from build123d import *

# Parameters (mm, degrees)
SKETCH_1_R      = 1.59
EXTRUDE_1_DEPTH = 1


with BuildPart() as part:
    # Эскиз1 → Бобышка-Вытянуть1 (new body)
    with BuildSketch(Plane(origin=(0, 0, 0), x_dir=(1, 0, 0), z_dir=(0, 1, 0))):
        with BuildLine():
            Line((-45.084998549, -11.549999236), (-45.084998549, -45.944999694))
            ThreePointArc((-45.084998549, -45.944999694), (-44.499026016, -47.35966253), (-43.084363181, -47.945635063))
            Line((-43.084363181, -47.945635063), (-11.549432233, -47.945635063))
            ThreePointArc((-11.549432233, -47.945635063), (-10.700904348, -47.594163453), (-10.349432233, -46.745635778))
            ThreePointArc((-10.349432233, -46.745635778), (-9.997959671, -45.897107024), (-9.149430707, -45.545634967))
            Line((-9.149430707, -45.545634967), (9.15056853, -45.545634967))
            ThreePointArc((9.15056853, -45.545634967), (9.999097494, -45.897107024), (10.350570056, -46.745635778))
            ThreePointArc((10.350570056, -46.745635778), (10.702042171, -47.594163453), (11.550570056, -47.945635063))
            Line((11.550570056, -47.945635063), (43.085566089, -47.945635063))
            ThreePointArc((43.085566089, -47.945635063), (44.499379352, -47.360014435), (45.08499998, -45.946201172))
            Line((45.08499998, -45.946201172), (45.08499998, -11.550001001))
            ThreePointArc((45.08499998, -11.550001001), (44.73352809, -10.70147331), (43.885000099, -10.350002145))
            ThreePointArc((43.885000099, -10.350002145), (43.03647086, -9.998530464), (42.684998454, -9.150001525))
            Line((42.684998454, -9.150001525), (42.684998454, 9.150001525))
            ThreePointArc((42.684998454, 9.150001525), (43.03647086, 9.998530464), (43.885000099, 10.350002145))
            ThreePointArc((43.885000099, 10.350002145), (44.733527178, 10.701472863), (45.08499962, 11.549999228))
            Line((45.08499962, 11.549999228), (45.08499962, 45.944999694))
            ThreePointArc((45.08499962, 45.944999694), (44.499213182, 47.359213257), (43.08499962, 47.944999694))
            Line((43.08499962, 47.944999694), (11.549999772, 47.944999694))
            ThreePointArc((11.549999772, 47.944999694), (10.701471635, 47.593527832), (10.349999772, 46.744999694))
            ThreePointArc((10.349999772, 46.744999694), (9.998527463, 45.896470478), (9.149998246, 45.544998168))
            Line((9.149998246, 45.544998168), (-9.149997176, 45.544998168))
            ThreePointArc((-9.149997176, 45.544998168), (-9.998526392, 45.896470478), (-10.349998702, 46.744999694))
            ThreePointArc((-10.349998702, 46.744999694), (-10.701470564, 47.593527832), (-11.549998702, 47.944999694))
            Line((-11.549998702, 47.944999694), (-43.084998549, 47.944999694))
            ThreePointArc((-43.084998549, 47.944999694), (-44.499212112, 47.359213257), (-45.084998549, 45.944999694))
            Line((-45.084998549, 45.944999694), (-45.084998549, 11.549999236))
            ThreePointArc((-45.084998549, 11.549999236), (-44.733526654, 10.701471175), (-43.884998501, 10.349999499))
            ThreePointArc((-43.884998501, 10.349999499), (-43.036470349, 9.998527823), (-42.684998454, 9.149999761))
            Line((-42.684998454, 9.149999761), (-42.684998454, -9.149999761))
            ThreePointArc((-42.684998454, -9.149999761), (-43.036470608, -9.998528446), (-43.884999384, -10.350000381))
            ThreePointArc((-43.884999384, -10.350000381), (-44.733526912, -10.701471799), (-45.084998549, -11.549999236))
        make_face()
        with Locations(Location((37.465001451, 42.865000306, 0), (0, 0, 270))):
            Circle(SKETCH_1_R, mode=Mode.SUBTRACT)
        with Locations(Location((40.005001451, -42.864999694, 0), (0, 0, 270))):
            Circle(SKETCH_1_R, mode=Mode.SUBTRACT)
        with Locations(Location((-40.004998549, -42.864999694, 0), (0, 0, 270))):
            Circle(SKETCH_1_R, mode=Mode.SUBTRACT)
        with Locations(Location((-36.194998549, 42.865000306, 0), (0, 0, 270))):
            Circle(SKETCH_1_R, mode=Mode.SUBTRACT)
    extrude(amount=EXTRUDE_1_DEPTH)


solid = part.part
Input: part model. Units: mm. Frame: model coordinates. Coordinates: 2 decimals unless noted, no trailing zeros. Order: outer loops, then holes, each group sorted by start corner. A loop starts at its lowest first (then second) coordinate and runs counter-clockwise, first axis right, second up.
1. Ray query, line 1 along Z through (x, y) = (40, 0.95) (3 decimals); line 2 along Z through (x, y) = (7, 0.9) (3 decimals); line 3 along Z through (x, y) = (41, 0.1) (3 decimals). Return the intervals inside material, ascending.
Checked values:
line 1: z = -47.945 to 41.275, 44.455 to 47.946
line 2: z = -45.545 to 45.546
line 3: z = -47.945 to 41.625, 44.105 to 47.946
2. Cut plane A-A, the plane x = -8. Return loops of the section in (y, z) (3 decimals), plus the area to 3 significant figures.
Checked values:
outline: (0, -45.545) - (1, -45.545) - (1, 45.546) - (0, 45.546) - close
area: 91.1 mm2
3. Cut plane B-B, the plane z = 4. Return loops of the section in (x, y) (3 decimals), plus the area to 3 significant figures.
Checked values:
outline: (-42.685, 0) - (42.685, 0) - (42.685, 1) - (-42.685, 1) - close
area: 85.4 mm2
4. Cut plane C-C, the plane y = 0.4. Count the separate pieces of the cut face and the enclosed holes in it, plus the area to 3 significant figures.
Checked values:
separate pieces: 1
enclosed holes: 4
area: 8,410 mm2
5. Contact query for flat-ended pins moving along their axis: P1, Ø3, axis at x = 40.01, z = 42.86, coming from the -Y side; P2, Ø0.5, axis at x = -2, y = 0.5, coming from the +Z side. Output: stop coordinate, or through.
Checked values:
P1: passes through
P2: stops at z = 45.55
6. Draft query along X for faces 1 (the flat face through (-1, 0, -1)), 2 (the cylindrical face through (38.8, 0.5, -42)), 3 (the cylindrical face through (41.346, 0.493, 43.72)), 4 (the cylindrical face through (44.515, 0.493, -47.344)). Return one class per face: +X half, -X half, draft (parallel to the pull), parting line (faces both ways), or undercut.
Checked values:
face 1: draft
face 2: undercut
face 3: undercut
face 4: +X half
